Can you work these out from the model? Positions are in its coordinate system, mm. Face numbers are marked on the shaded views. A direction names the side the tool comes from. Coordinates: 2 decimals unless noted, no trailing zeros. Order: outer loops, then holes, each group sorted by start corner. A loop starts at its lowest first (then second) coordinate and runs counter-clockwise, first axis right, second up. Notation, with made-up numbers: (59, 44) - (78, 44) arc R16 ccw to (78, 60) - close; hole circle Ø1 at (17.5, 1). An arc over 180 degrees is marked (long way). Use a Markdown table: item, result. Add a question column.
(1) On a 3-axis mill with a long thin cutter (end or side, diameter ignored), from which of +Z, -Z, +X, -X, +Y, -Y can I reach the whole of each face in a straight line? I mean the marked faces 1, 2, 3 and 4. Say none if no direction works.
(2) I want a section at A-A (z = 16.5). List the corners of the cut face in (x, y) for me, and give its area (3 significant figures).
(3) If I drill on L1, parallel to Y at x = -13, z = -37; L2, parallel to Z at x = -11, y = -7.5; L3, parallel to X at y = -5, z = 41.5, over which ranges is the centre line in solid material (lowest first)? Write a range as [from, to].
(4) I want a section at C-C (x = 13.5). List the corners of the cut face in (y, z) for me, and give its area (3 significant figures).
(5) For pin 1 Ø3 at (x, y) = (34.5, -12.5) entering from -Z; pin 2 Ø1 at (y, z) = (-12.5, 18) entering from +X (3 decimals); pin 3 Ø6 at (y, z) = (-6, 29.5) entering from +X, each with a flat end and sliding along its axis, tell me the tip position at first contact or that it passes through.
(6) I want a section at B-B (y = -8.5). List the corners of the cut face in (x, z) for me, and give its area (3 significant figures).
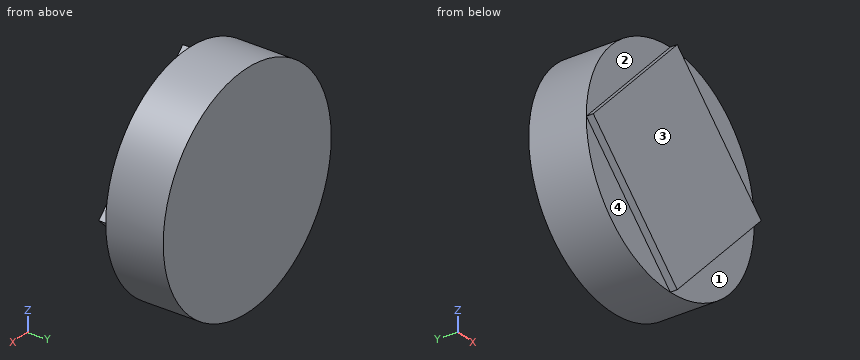
```python
from build123d import *

# Parameters (mm, degrees)
F0_R     = 49.267776
F1_DEPTH = 25.4
F3_DEPTH = 3.0734


with BuildPart() as f1:
    # F0 (on Front) → F1 (new body)
    with BuildSketch(Plane.XZ):
        Circle(F0_R)
    extrude(amount=F1_DEPTH)

    # F2 (on face) → F3 (join)
    with BuildSketch(Plane.XZ.offset(25.4)):
        Polygon((49.267776, 0), (0, 49.267776), (-49.267776, 0), (0, -49.267776), align=None)
    extrude(amount=F3_DEPTH)


solid = f1.part
```
Answers follow:
| question | item | result |
|---|---|---|
| 1 | face 1 | -Z, +X, -Y |
| 1 | face 2 | +Z, -X, -Y |
| 1 | face 3 | +Z, -Z, +X, -X, -Y |
| 1 | face 4 | -Z, -X, -Y |
| 2 | outline | (-46.42, -25.4) - (-32.77, -25.4) - (-32.77, -28.47) - (32.77, -28.47) - (32.77, -25.4) - (46.42, -25.4) - (46.42, 0) - (-46.42, 0) - close |
| 2 | area | 2,560 mm² |
| 3 | L1 | y = [-25.4, 0] |
| 3 | L2 | z = [-48.02, 48.02] |
| 3 | L3 | x = [-26.55, 26.55] |
| 4 | outline | (-28.47, -35.77) - (-25.4, -35.77) - (-25.4, -47.38) - (0, -47.38) - (0, 47.38) - (-25.4, 47.38) - (-25.4, 35.77) - (-28.47, 35.77) - close |
| 4 | area | 2,630 mm² |
| 5 | pin 1 | stops at z = -36.58 |
| 5 | pin 2 | stops at x = 46.055 |
| 5 | pin 3 | stops at x = 41.53 |
| 6 | outline | circle Ø98.54 at (0, 0) |
| 6 | area | 7,630 mm² |
